from build123d import *

# Parameters (mm, degrees)
SKETCH_2_W           = 80
SKETCH_2_H           = 16
EXTRUDE_1_DEPTH      = 8
SKETCH_5_R           = 1.55
CUT_EXTRUDE_3_DEPTH  = 82.975606128
CUT_EXTRUDE_4_DEPTH  = 82.975606128
SKETCH_8_W           = 3
SKETCH_8_H           = 16
CUT_EXTRUDE_5_DEPTH  = 4
SKETCH_9_R           = 0.5
CUT_EXTRUDE_6_DEPTH  = 82.975606128
CUT_EXTRUDE_7_DEPTH  = 2
CUT_EXTRUDE_8_DEPTH  = 82.975606128
SKETCH_12_W          = 5.7
SKETCH_12_H          = 2.5
CUT_EXTRUDE_9_DEPTH  = 2
SKETCH_13_W          = 2
SKETCH_13_H          = 14
CUT_EXTRUDE_10_DEPTH = 0.5


with BuildPart() as part:
    # 草图2 → 凸台-拉伸1 (new body)
    with BuildSketch(Plane.XY):
        with Locations((40, 8)):
            Rectangle(SKETCH_2_W, SKETCH_2_H)
        with BuildLine():
            ThreePointArc((11.048765244, 7.9), (7, 11.85), (2.951234756, 7.9))
            ThreePointArc((2.951234756, 7.9), (7, 3.95), (11.048765244, 7.9))
        make_face(mode=Mode.SUBTRACT)
        with BuildLine():
            ThreePointArc((77.048765244, 7.9), (73, 11.85), (68.951234756, 7.9))
            ThreePointArc((68.951234756, 7.9), (73, 3.95), (77.048765244, 7.9))
        make_face(mode=Mode.SUBTRACT)
    extrude(amount=EXTRUDE_1_DEPTH)

    # 草图5 → 切除-拉伸3 (cut, through all)
    with BuildSketch(Plane.XY.offset(8)):
        with Locations((48, 9.8)):
            Circle(SKETCH_5_R)
        with Locations((32, 9.8)):
            Circle(SKETCH_5_R)
    extrude(amount=-CUT_EXTRUDE_3_DEPTH, mode=Mode.SUBTRACT)

    # 草图6 → 切除-拉伸4 (cut, through all)
    with BuildSketch(Plane.XY.offset(8)):
        with BuildLine():
            Line((3.102244235, 8.9), (0, 8.9))
            Line((0, 8.9), (0, 6.9))
            Line((0, 6.9), (3.102244235, 6.9))
            ThreePointArc((3.102244235, 6.9), (2.995402762, 7.395267856), (2.951234756, 7.9))
            ThreePointArc((2.951234756, 7.9), (2.995402762, 8.404732144), (3.102244235, 8.9))
        make_face()
        with BuildLine():
            ThreePointArc((60, 5.4), (61.224744871, 5.81886117), (61.936491673, 6.9))
            Line((61.936491673, 6.9), (64, 6.9))
            ThreePointArc((64, 6.9), (65, 7.9), (64, 8.9))
            Line((64, 8.9), (60, 8.9))
            ThreePointArc((60, 8.9), (58.775255129, 8.48113883), (58.063508327, 7.4))
            Line((58.063508327, 7.4), (21.936491673, 7.4))
            ThreePointArc((21.936491673, 7.4), (21.224744871, 8.48113883), (20, 8.9))
            Line((20, 8.9), (16, 8.9))
            ThreePointArc((16, 8.9), (15, 7.9), (16, 6.9))
            Line((16, 6.9), (18.063508327, 6.9))
            ThreePointArc((18.063508327, 6.9), (18.775255129, 5.81886117), (20, 5.4))
            Line((20, 5.4), (60, 5.4))
        make_face()
        with BuildLine():
            Line((76.897755765, 6.9), (80, 6.9))
            Line((80, 6.9), (80, 8.9))
            Line((80, 8.9), (76.897755765, 8.9))
            ThreePointArc((76.897755765, 8.9), (77.004597237, 8.404732144), (77.048765244, 7.9))
            ThreePointArc((77.048765244, 7.9), (77.004597237, 7.395267856), (76.897755765, 6.9))
        make_face()
        with BuildLine():
            Line((67, 6.9), (69.102244235, 6.9))
            ThreePointArc((69.102244235, 6.9), (68.995402763, 7.395267856), (68.951234756, 7.9))
            ThreePointArc((68.951234756, 7.9), (68.995402763, 8.404732144), (69.102244235, 8.9))
            Line((69.102244235, 8.9), (67, 8.9))
            ThreePointArc((67, 8.9), (66, 7.9), (67, 6.9))
        make_face()
        with BuildLine():
            Line((13, 8.9), (10.897755764, 8.9))
            ThreePointArc((10.897755764, 8.9), (11.004597237, 8.404732144), (11.048765244, 7.9))
            ThreePointArc((11.048765244, 7.9), (11.004597237, 7.395267856), (10.897755764, 6.9))
            Line((10.897755764, 6.9), (13, 6.9))
            ThreePointArc((13, 6.9), (14, 7.9), (13, 8.9))
        make_face()
    extrude(amount=-CUT_EXTRUDE_4_DEPTH, mode=Mode.SUBTRACT)

    # 草图8 → 切除-拉伸5 (cut)
    with BuildSketch(Plane.XY.offset(8)):
        with Locations((40, 8)):
            Rectangle(SKETCH_8_W, SKETCH_8_H)
    extrude(amount=-CUT_EXTRUDE_5_DEPTH, mode=Mode.SUBTRACT)

    # 草图9 → 切除-拉伸6 (cut, through all)
    with BuildSketch(Plane.XY.offset(8)):
        with Locations((37.65, 1.5)):
            Circle(SKETCH_9_R)
        with Locations((42.35, 1.5)):
            Circle(SKETCH_9_R)
        with BuildLine():
            Line((38.5, 2), (38.5, 0))
            Line((38.5, 0), (42.85, 0))
            Line((42.85, 0), (42.85, 1.5))
            ThreePointArc((42.85, 1.5), (41.996446609, 1.146446609), (42.35, 2))
            Line((42.35, 2), (38.5, 2))
        make_face()
        with BuildLine():
            Line((37.15, 1.5), (37.15, 0))
            Line((37.15, 0), (38.5, 0))
            Line((38.5, 0), (38.5, 2))
            Line((38.5, 2), (37.65, 2))
            ThreePointArc((37.65, 2), (38.003553391, 1.853553391), (38.15, 1.5))
            ThreePointArc((38.15, 1.5), (37.65, 1), (37.15, 1.5))
        make_face()
    extrude(amount=-CUT_EXTRUDE_6_DEPTH, mode=Mode.SUBTRACT)

    # 草图10 → 切除-拉伸7 (cut)
    with BuildSketch(Plane.XY.offset(8)):
        with BuildLine():
            Line((37, 10.5), (43, 10.5))
            ThreePointArc((43, 10.5), (47, 6.5), (43, 2.5))
            Line((43, 2.5), (37, 2.5))
            ThreePointArc((37, 2.5), (33, 6.5), (37, 10.5))
        make_face()
    extrude(amount=-CUT_EXTRUDE_7_DEPTH, mode=Mode.SUBTRACT)

    # 草图11 → 切除-拉伸8 (cut, through all)
    with BuildSketch(Plane.XY.offset(8)):
        with BuildLine():
            Line((37, 5.4), (43, 5.4))
            ThreePointArc((43, 5.4), (44.75, 7.15), (43, 8.9))
            Line((43, 8.9), (37, 8.9))
            ThreePointArc((37, 8.9), (35.25, 7.15), (37, 5.4))
        make_face()
    extrude(amount=-CUT_EXTRUDE_8_DEPTH, mode=Mode.SUBTRACT)

    # 草图12 → 切除-拉伸9 (cut)
    with BuildSketch(Plane.XY.offset(8)):
        with Locations((40, 1.25)):
            Rectangle(SKETCH_12_W, SKETCH_12_H)
    extrude(amount=-CUT_EXTRUDE_9_DEPTH, mode=Mode.SUBTRACT)

    # 草图13 → 切除-拉伸10 (cut)
    with BuildSketch(Plane.XY.offset(4)):
        with Locations((40, 9)):
            Rectangle(SKETCH_13_W, SKETCH_13_H)
    extrude(amount=-CUT_EXTRUDE_10_DEPTH, mode=Mode.SUBTRACT)


solid = part.part
Here's how the part is built. I have some questions about the finished solid (model axes, mm). A direction names the side the tool comes from. Round coordinates to 2 decimals unless told otherwise and drop trailing zeros. Loops run counter-clockwise (first coordinate to the right, second up) from the corner with the lowest first, then second, coordinate; pieces in that order, holes last. Notation, with made-up numbers: M -23,6 L 9,6 A23 ccw 9,38 Z; hole C 29,63 d5. An arc over 180 degrees is marked long. Write each question's results on one line, items separated by ' | '. Start each with the question number.
(1) If I drill on probe 1 along Y at (x, z) = (48, 4.75); probe 2 along X at (y, z) = (10.75, 2); probe 3 along Y at (x, z) = (24, 4.25), over which ranges is the centre line in solid material (lowest first)? Write a range as from..to.
(2) Will these pins go through, and if not, where does the flat tip stop? P1, Ø0.6, axis at x = 41, y = 11, coming from the +Z side; P2, Ø0.8, axis at x = 42, z = 7, coming from the -Y side.
(3) I want a section at B-B (y = 13). Please give me the cut outline in (x, z).
(4) I want a section at A-A (x = 53). Please give me the cut outline in (y, z), then the cut area to 3 significant figures.
(5) Thinking about a two-plate mould opening in Y: for faces 1 (the flat face through (2, 8.9, 4)), 2 (the flat face through (38.5, 4, 5)), which applies, pulls with the +Y half, pulls with the -Y half, needs draft (parallel to the pull), parting line crosses it, or undercut?
(6) I want a section at C-C (z = 7). State how many separate pieces and enclosed holes the cut face has, then the cut area to 3 significant figures.
(7) On a 3-axis mill with a long thin cutter (end or side, diameter ignored), from which of +Z, -Z, +X, -X, +Y, -Y can I reach the whole of each face in a straight line? I mean faces 3 (the flat face through (12, 6.9, 4)), 4 (the cylindrical face through (45.4, 3.3, 7)), 5 (the flat face through (41.5, 4, 5)), 6 (the cylindrical face through (65, 7.9, 4.1)). Say none if no direction works.
Solved:
1) probe 1: y = 0..5.4, 7.4..8.25, 11.35..16 | probe 2: x = 0..4.23, 9.77..30.78, 33.22..46.78, 49.22..70.23, 75.77..80 | probe 3: y = 0..5.4, 7.4..16
2) P1: stops at z = 4 | P2: stops at y = 10.5
3) outline: M 0,0 L 80,0 L 80,8 L 41.5,8 L 41.5,4 L 41,4 L 41,3.5 L 39,3.5 L 39,4 L 38.5,4 L 38.5,8 L 0,8 Z
4) outline: M 0,0 L 5.4,0 L 5.4,8 L 0,8 Z; M 7.4,0 L 16,0 L 16,8 L 7.4,8 Z | area: 112 mm²
5) face 1: undercut | face 2: needs draft
6) separate pieces: 2 | enclosed holes: 2 | area: 933 mm²
7) face 3: +Z, -Z, -X | face 4: +Z | face 5: +Z, +Y, -Y | face 6: +Z, -Z
